CAD build for the part. Positions are in the model's coordinates, mm. Face numbers are marked on the shaded views. Round coordinates to 2 decimals unless told otherwise and drop trailing zeros. Order: outer loops, then holes, each group sorted by start corner. A loop starts at its lowest first (then second) coordinate and runs counter-clockwise, first axis right, second up. Notation, with made-up numbers: (-14.75, -30) - (-2.75, -30) arc R19 cw to (-2.75, -8) - close; hole circle Ø3 at (-13.5, 84.5). An arc over 180 degrees is marked (long way). Write item = value, one per line.
from build123d import *

# Parameters (mm, degrees)
SKETCH1_W           = 50
SKETCH1_H           = 120
BOSS_EXTRUDE1_DEPTH = 20
SKETCH11_W          = 10
SKETCH11_H          = 5
BOSS_EXTRUDE5_DEPTH = 15
SKETCH13_R          = 1
CUT_EXTRUDE3_DEPTH  = 10
SKETCH14_W          = 19.8
SKETCH14_H          = 36
CUT_EXTRUDE4_DEPTH  = 9.3
SKETCH15_W          = 19.8
SKETCH15_H          = 2.5
CUT_EXTRUDE5_DEPTH  = 7.1


with BuildPart() as part:
    # Sketch1 → Boss-Extrude1 (new body)
    with BuildSketch(Plane(origin=(0, 0, 0), x_dir=(1, 0, 0), z_dir=(0, 1, 0))):
        with Locations((-3.706441645, 54.181126694)):
            Rectangle(SKETCH1_W, SKETCH1_H)
    extrude(amount=BOSS_EXTRUDE1_DEPTH)

    # Sketch11 → Boss-Extrude5 (add)
    with BuildSketch(Plane(origin=(0, 20, 0), x_dir=(1, 0, 0), z_dir=(0, 1, 0))):
        with Locations((-3.706441645, 1.681126694)):
            Rectangle(SKETCH11_W, SKETCH11_H)
    extrude(amount=BOSS_EXTRUDE5_DEPTH)

    # Sketch13 → Cut-Extrude3 (cut)
    with BuildSketch(Plane(origin=(0, 0, -4.181126694), x_dir=(-1, 0, 0), z_dir=(0, 0, -1))):
        with Locations((3.706441645, 30)):
            Circle(SKETCH13_R)
    extrude(amount=-CUT_EXTRUDE3_DEPTH, mode=Mode.SUBTRACT)

    # Sketch14 → Cut-Extrude4 (cut)
    with BuildSketch(Plane(origin=(0, 20, 0), x_dir=(1, 0, 0), z_dir=(0, 1, 0))):
        with Locations((-3.331441645, 72.181126694)):
            Rectangle(SKETCH14_W, SKETCH14_H)
    extrude(amount=-CUT_EXTRUDE4_DEPTH, mode=Mode.SUBTRACT)

    # Sketch15 → Cut-Extrude5 (cut)
    with BuildSketch(Plane(origin=(0, 10.7, 0), x_dir=(1, 0, 0), z_dir=(0, 1, 0))):
        with Locations((-3.331441645, 62.431126694)):
            Rectangle(SKETCH15_W, SKETCH15_H)
    extrude(amount=-CUT_EXTRUDE5_DEPTH, mode=Mode.SUBTRACT)


solid = part.part
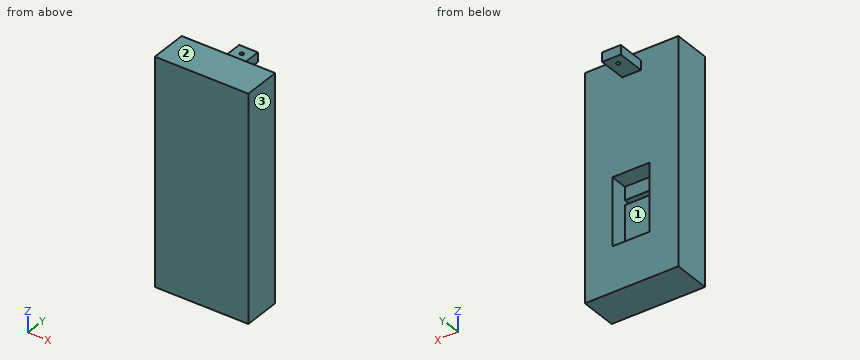
(1) Probe line 1 along Z through (x, y) = (3.5, 5.5); line 2 along Y through (x, z) = (-17, -84); line 3 along Z through (x, y) = (-3.5, 33). List the from-to ranges inside material, lowest first.
Solved:
line_1 = -114.18 to -63.68, -61.18 to 5.82
line_2 = 0 to 20
line_3 = -4.18 to 0.82
(2) Band-saw the part on A-A on z = -65.5. List the corners of the cut face in (x, y), plus the area to 3 significant figures.
Solved:
outline = (-28.71, 0) - (21.29, 0) - (21.29, 20) - (6.57, 20) - (6.57, 10.7) - (-13.23, 10.7) - (-13.23, 20) - (-28.71, 20) - close
area = 816 mm²
(3) Drop flat-ended pins along their axis: pin 1 (25 mm diameter, centred on x = 6, z = -33, fed in from +Y); pin 2 (3 mm diameter, centred on x = 8, z = -87, fed in from -Y); pin 3 (8 mm diameter, centred on x = -3, y = 25.5, fed in from -Z); pin 4 (5.5 mm diameter, centred on x = -8.5, z = -59.5, fed in from +Y). Give the stop position or say it passes through.
Solved:
pin_1 = 20
pin_2 = 0
pin_3 = -4.18
pin_4 = 10.7
(4) Band-saw the part on B-B on x = -6. List the corners of the cut face in (y, z), plus the area to 3 significant figures.
Solved:
outline = (0, -114.18) - (20, -114.18) - (20, -90.18) - (10.7, -90.18) - (10.7, -63.68) - (3.6, -63.68) - (3.6, -61.18) - (10.7, -61.18) - (10.7, -54.18) - (20, -54.18) - (20, -4.18) - (35, -4.18) - (35, 0.82) - (20, 0.82) - (20, 5.82) - (0, 5.82) - close
area = 2,120 mm²
(5) Band-saw the part on D-D on x = 9. List the corners of the cut face in (y, z), plus the area to 3 significant figures.
Solved:
outline = (0, -114.18) - (20, -114.18) - (20, 5.82) - (0, 5.82) - close
area = 2,400 mm²
(6) Pull direction X, two halves, no side cores. Call the marked faces 1, 2 and 3: released by +X, released by -X, zero draft, split by the parting line, or undercut.
Solved:
face_1 = undercut
face_2 = zero draft
face_3 = released by +X
(7) Band-saw the part on C-C on z = -91.5. List the corners of the cut face in (x, y), plus the area to 3 significant figures.
Solved:
outline = (-28.71, 0) - (21.29, 0) - (21.29, 20) - (-28.71, 20) - close
area = 1,000 mm²
